The model under review builds one solid part; all positions refer to its coordinate system, in mm. Face numbers are marked on the shaded views. A direction names the side the tool comes from. Coordinates: 2 decimals unless noted, no trailing zeros. Loops run counter-clockwise (first coordinate to the right, second up) from the corner with the lowest first, then second, coordinate; pieces in that order, holes last. Notation, with made-up numbers: (68.5, 63) - (91.5, 63) arc R20 ccw to (91.5, 88) - close; hole circle Ø1 at (58.25, -8). An arc over 180 degrees is marked (long way). One line per item, written item: value. Start each with the question number.
1. We need section C-C, the plane x = 4.25. Give the boundary of the cut face in (y, z), then the cut area to 3 significant figures.
2. We need section D-D, the plane z = -4. Give the boundary of the cut face in (x, y).
3. We need section B-B, the plane y = 2.15. Give the boundary of the cut face in (x, z), then the cut area to 3 significant figures.
4. We need section A-A, the plane z = -3. Give the boundary of the cut face in (x, y), then the cut area to 3 significant figures.
5. For the marked faces 4, 5 and 6, list the 3-axis set-ups (+Z, -Z, +X, -X, +Y, -Y) from which the entire face can be reached by the end or side of a thin tool; tool diameter is ignored.
6. To check wall thickness, follow line 1 (Y direction, x = 2.5, z = -6.75); line 2 (X direction, y = 0.65, z = -3.75); line 3 (Z direction, x = 5.5, y = -1.1). State the ranges of each line that lie inside material, in increasing order.
7. Mouldability with a two-part tool opening along X and no side actions: class the marked faces 1, 2 and 3 as +X half, -X half, draft (parallel to the pull), parting line (faces both ways), or undercut.
8. Insertion check: P1, Ø4, axis at x = 4, z = -3.75, coming from the -Y side; P2, Ø1, axis at x = 4.5, y = -1, coming from the +Z side. Each pin has a flat end and moves straight along its axis. Give the tip position at first contact, or say it passes through.
from build123d import *

# Parameters (mm, degrees)
SKETCH1_W               = 8
SKETCH1_H               = 8
BOSS_EXTRUDE1_DEPTH     = 3
CUT_EXTRUDE1_DEPTH      = 12.704699911
CUT_EXTRUDE1_DEPTH_BACK = 12.704699911
CUT_EXTRUDE2_DEPTH      = 11
SKETCH4_R               = 1.8
CUT_EXTRUDE3_DEPTH      = 0.8
SKETCH5_W               = 8
SKETCH5_H               = 1
BOSS_EXTRUDE2_DEPTH     = 2
FILLET1_R               = 4
CUT_EXTRUDE4_DEPTH      = 0.4


with BuildPart() as part:
    # Sketch1 → Boss-Extrude1 (new body)
    with BuildSketch(Plane(origin=(0, 0, 0), x_dir=(1, 0, 0), z_dir=(0, 1, 0))):
        with Locations((4, 4)):
            Rectangle(SKETCH1_W, SKETCH1_H)
    extrude(amount=BOSS_EXTRUDE1_DEPTH)

    # Sketch2 → Cut-Extrude1 (cut, two sides: drawn at the far end of the back side and taken through both)
    with BuildSketch(Plane.XY.offset(-CUT_EXTRUDE1_DEPTH_BACK)):
        Polygon((0, 0), (0.6, 3), (0, 3), align=None)
        Polygon((8, 0), (7.4, 3), (8, 3), align=None)
    extrude(amount=CUT_EXTRUDE1_DEPTH + CUT_EXTRUDE1_DEPTH_BACK, mode=Mode.SUBTRACT)

    # Sketch3 → Cut-Extrude2 (cut)
    with BuildSketch(Plane(origin=(0, 0, 0), x_dir=(0, 0, -1), z_dir=(1, 0, 0))):
        Polygon((0, 0), (0.6, 3), (0, 3), align=None)
        Polygon((8, 3), (7.4, 3), (8, 0), align=None)
    extrude(amount=CUT_EXTRUDE2_DEPTH, mode=Mode.SUBTRACT)

    # Sketch4 → Cut-Extrude3 (cut)
    with BuildSketch(Plane.XZ):
        with Locations(Location((4, -3.75, 0), (0, 0, 270))):
            Circle(SKETCH4_R)
    extrude(amount=-CUT_EXTRUDE3_DEPTH, mode=Mode.SUBTRACT)

    # Sketch5 → Boss-Extrude2 (add)
    with BuildSketch(Plane.XZ):
        with Locations((4, -7.5)):
            Rectangle(SKETCH5_W, SKETCH5_H)
    extrude(amount=BOSS_EXTRUDE2_DEPTH)

    # Fillet1
    # the kernel refuses this fillet: 4 mm, written as the material it takes off along each edge
    with BuildSketch(Plane(origin=(8, -2, -16.660254038), x_dir=(0, 1, 0), z_dir=(0, 0, 1)), Plane(origin=(0, -2, 1.660254038), x_dir=(0, 1, 0), z_dir=(0, 0, -1))) as fillet1_piece_1:
        with BuildLine():
            CenterArc((4, 3.464101615), FILLET1_R, 180, 60)
            Line((0, 3.464101615), (-0.08, 3.464101615))
            Line((-0.08, 3.464101615), (-0.08, 0))
            Line((-0.08, 0), (0, -0.08))
            ThreePointArc((0, -0.08), (1, -0.08), (1.96, -0.069282032))
            Line((1.96, -0.069282032), (2, 0))
        make_face()
    extrude(amount=18.320508076, mode=Mode.SUBTRACT)

    # Sketch6 → Cut-Extrude4 (cut)
    with BuildSketch(Plane(origin=(0, 3, 0), x_dir=(1, 0, 0), z_dir=(0, 1, 0))):
        Polygon((2.136477101, 1.987434605), (3.507470691, 4.106024349), (2.290323255, 5.987434605), (3.189361717, 5.987434605), (3.956989922, 4.800735887), (4.724618127, 5.987434605), (5.623656589, 5.987434605), (4.406509153, 4.106024349), (5.777502742, 1.987434605), (4.878464281, 1.987434605), (3.956989922, 3.41131281), (3.035515563, 1.987434605), align=None)
    extrude(amount=-CUT_EXTRUDE4_DEPTH, mode=Mode.SUBTRACT)


solid = part.part
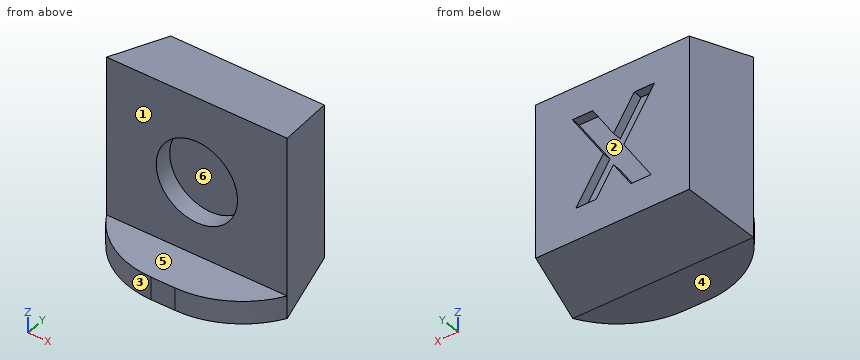
Findings below:
1. outline: (-2, -8) - (0, -8) - (3, -7.4) - (3, -5.25) - (2.6, -5.25) - (2.6, -2.96) - (3, -2.96) - (3, -0.6) - (0, 0) - (0, -1.97) - (0.8, -1.97) - (0.8, -5.53) - (0, -5.53) - (0, -7) - (-2, -7) - close
1. area: 20.4 mm2
2. outline: (0, 0) - (2.22, 0) - (2.22, 0.8) - (5.78, 0.8) - (5.78, 0) - (8, 0) - (7.4, 3) - (4.48, 3) - (4.48, 2.6) - (3.44, 2.6) - (3.44, 3) - (0.6, 3) - close
3. outline: (0.43, -7.57) - (7.57, -7.57) - (7.57, -0.43) - (0.43, -0.43) - close
3. area: 51.0 mm2
4. outline: (0, 0) - (2.36, 0) - (2.36, 0.8) - (5.64, 0.8) - (5.64, 0) - (8, 0) - (7.4, 3) - (5.12, 3) - (5.12, 2.6) - (4.22, 2.6) - (4.22, 3) - (3.69, 3) - (3.69, 2.6) - (2.79, 2.6) - (2.79, 3) - (0.6, 3) - close
4. area: 18.9 mm2
5. face 4: -Z, +X, -X, +Y, -Y
5. face 5: +Z, +X, -X, -Y
5. face 6: -Y
6. line 1: 0 to 3
6. line 2: 0.13 to 2.2, 5.8 to 7.87
6. line 3: -8 to -7
7. face 1: draft
7. face 2: undercut
7. face 3: -X half
8. P1: y = 0
8. P2: z = -7
